Source: CAD feature listing. Evaluate the final solid. Frame: model axes, mm. A direction names the side the tool comes from. Give positions to 0.01 mm unless a question says otherwise; leave off trailing zeros. Order: outer loops, then holes, each group sorted by start corner. A loop starts at its lowest first (then second) coordinate and runs counter-clockwise, first axis right, second up.
1) Section C-C, the plane x = 1160.5. Return loops of the section in (y, z).
2) Material intervals for line 1 (Z direction, x = 1614, y = 194.5); line 2 (Y direction, x = 1615, z = 150), sorted ascending.
3) Section A-A, the plane y = 341. Return loops of the section in (x, z), plus the area to 3 significant figures.
4) First-contact query: P1, Ø1.5, axis at x = 790, z = 652.5, coming from the -Y side. Flat tip, straight axial feed; report the tip coordinate or a pass-through.
5) Access query for faces 1 (the face through (0, 611, 368)), 2 (the face through (100, 296, 51)), 3 (the face through (51, 296, 100)). Directions: +Z, -Z, +X, -X, +Y, -Y. A direction counts if a zero-diameter tool reaches every point of the face in a straight line with its end or side. Return the directions, or none.
6) Draft query along Z for faces 4 (the face through (846, 611, 0)), 5 (the face through (1600, 304, 691)), 6 (the face through (846, 611, 740)), 7 (the face through (1651, 296, 100)). Return one class per face: released by +Z, released by -Z, zero draft, split by the parting line, or undercut.
7) Section D-D, the plane z = 565.5. Return loops of the section in (x, y).
8) Section B-B, the plane z = 71.5. Return loops of the section in (x, y).
Autodesk Inventor part; units mm, degrees
ref_plane "YZ Plane" through (0, 0, 0) normal (1, 0, 0) x (0, 1, 0)
ref_plane "XZ Plane" through (0, 0, 0) normal (0, 1, 0) x (-1, 0, 0)
ref_plane "XY Plane" through (0, 0, 0) normal (0, 0, 1) x (1, 0, 0)
sketch "Sketch1" plane through (0, 0, 0) normal (0, 0, 1) x (1, 0, 0)
  point P0 (0, 0)
sketch "Sketch2" plane through (0, 0, 0) normal (0, 0, 1) x (1, 0, 0)
  line L0 (0, 0) -> (1700, 0)
  line L1 (1700, 0) -> (1700, 700)
  line L2 (1700, 700) -> (0, 700)
  line L3 (0, 700) -> (0, 0)
  dimension "d0" = 700
  dimension "d1" = 1700
extrude "Extrusion1" add sketch "Sketch2" along normal blind 740
sketch "Sketch3" plane through (0, 0, 740) normal (0, 0, 1) x (1, 0, 0)
  line L0 (1600, 0) -> (100, 0)
  line L1 (100, 0) -> (100, 600)
  line L2 (100, 600) -> (1600, 600)
  line L3 (1600, 600) -> (1600, 0)
  line L4 (1700, 700) -> (0, 700)
  line L5 (1700, 0) -> (1700, 700)
  line L6 (0, 700) -> (0, 0)
  dimension "d4" = 100
  dimension "d5" = 100
  dimension "d6" = 100
extrude "Extrusion2" cut sketch "Sketch3" against normal blind 740
sketch "Sketch4" plane through (1700, 0, 0) normal (1, 0, 0) x (0, 0, -1)
  line L0 (0, 0) -> (-740, 0)
  line L1 (-640, 0) -> (-100, 0)
  line L2 (-100, 0) -> (-100, 600)
  line L3 (-100, 600) -> (-640, 600)
  line L4 (-640, 600) -> (-640, 0)
  line L5 (0, 700) -> (-740, 700)
  line L6 (-740, 600) -> (-740, 0)
  line L7 (0, 0) -> (0, 700)
  dimension "d9" = 100
  dimension "d10" = 100
  dimension "d11" = 100
extrude "Extrusion3" cut sketch "Sketch4" against normal blind 4000
properties part number "computerBottom" material "Aluminum 6061, Welded"
From the geometry:
1. outline: (600, 0) - (700, 0) - (700, 740) - (600, 740) - close
2. line 1: z = 0 to 100, 640 to 740
2. line 2: y = 600 to 700
3. outline: (0, 0) - (100, 0) - (100, 100) - (0, 100) - close; (0, 640) - (100, 640) - (100, 740) - (0, 740) - close; (1600, 0) - (1700, 0) - (1700, 100) - (1600, 100) - close; (1600, 640) - (1700, 640) - (1700, 740) - (1600, 740) - close
3. area: 40,000 mm2
4. P1: stops at y = 600
5. face 1: +Z, -Z, -X, +Y, -Y
5. face 2: +Z, -Z, -Y
5. face 3: +X, -X, -Y
6. face 4: released by -Z
6. face 5: zero draft
6. face 6: released by +Z
6. face 7: undercut
7. outline: (0, 600) - (1700, 600) - (1700, 700) - (0, 700) - close
8. outline: (0, 0) - (100, 0) - (100, 600) - (1600, 600) - (1600, 0) - (1700, 0) - (1700, 700) - (0, 700) - close
